The figure shows three views and two pictorial views of one solid part (mm, origin at its lowest corner). Answer the questions. A direction names the side the tool comes from. Coordinates: 2 decimals unless noted, no trailing zeros. Loops run counter-clockwise (first coordinate to the right, second up) from the corner with the lowest first, then second, coordinate; pieces in that order, holes last. Notation, with made-up numbers: M 70,54.5 L 106,54.5 A24 cw 106,92.5 Z; hole C 58.5,69.25 d5. An arc over 180 degrees is marked long. Answer as a JSON object with one key per item and string values. Group by question number.
1. A cutting plane is placed at A-A on x = 10. Give the vertices of the cut face in (y, z), and give its area (3 significant figures).
2. A cutting plane is placed at B-B on z = 2.75. Give the vertices of the cut face in (x, y).
3. For the marked faces 1 and 2, determine the directions among +Z, -Z, +X, -X, +Y, -Y from which every point of the face is accessible in a straight line to the end or side of a thin tool.
4. A cutting plane is placed at D-D on x = 12.5. Give the vertices of the cut face in (y, z).
5. Given pin 1 (6 mm diameter, centred on x = 7.5, y = 23, fed in from -Z); pin 2 (1 mm diameter, centred on x = 4, z = 21.5, fed in from +Y); pin 3 (3 mm diameter, centred on x = 13, y = 40, fed in from +Z), each flat-ended and moving along its own axis, determine where each tip first touches the part or whether it passes through.
6. A cutting plane is placed at C-C on y = 32. Give the vertices of the cut face in (x, z), and give its area (3 significant figures).
7. Straight lines are drawn through the part: L1, parallel to Z at x = 11, y = 3; L2, parallel to X at y = 35, z = 6.75; L3, parallel to X at y = 36, z = 5.25. For each, find the intervals that lie inside material, in ascending order.
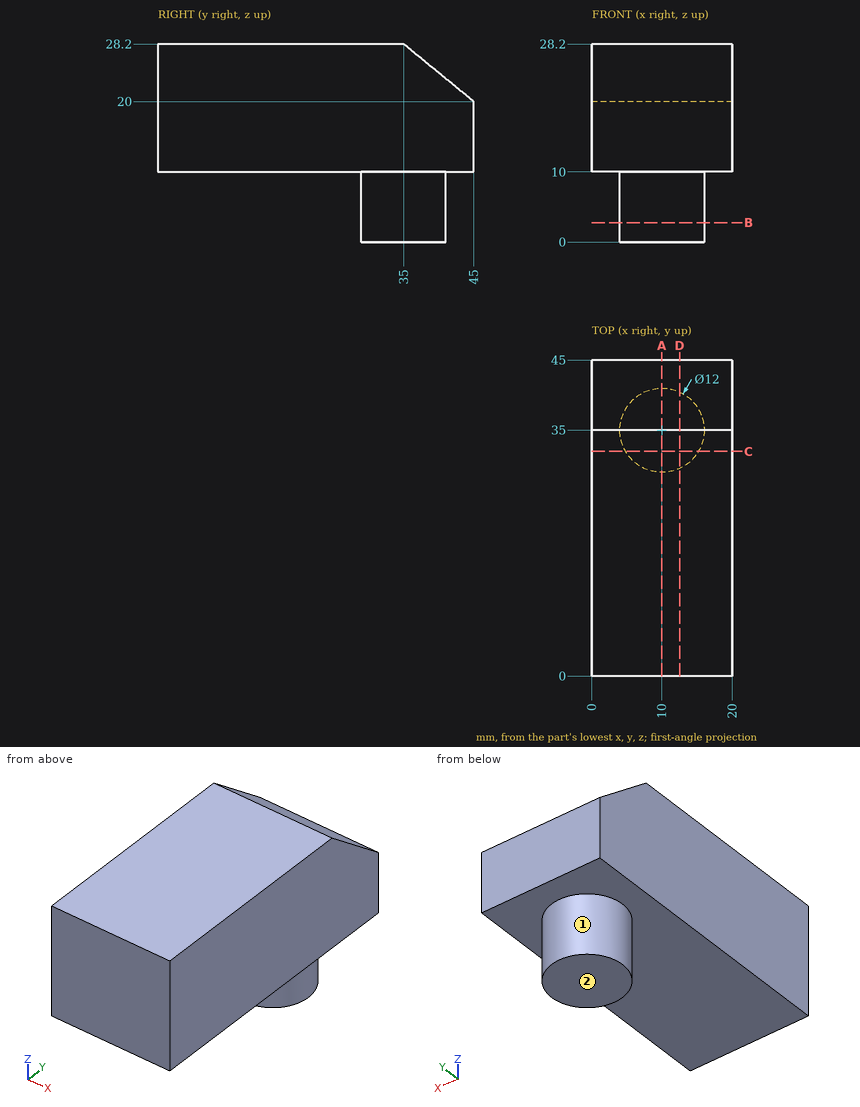
From the geometry:
{
 "1": {"outline": "M 0,10 L 29,10 L 29,0 L 41,0 L 41,10 L 45,10 L 45,20 L 35,28.2 L 0,28.2 Z", "area": "898 mm²"},
 "2": {"outline": "C 10,35 d12"},
 "3": {"face 1": "-Z", "face 2": "-Z, +X, -X, +Y, -Y"},
 "4": {"outline": "M 0,10 L 29.55,10 L 29.55,0 L 40.45,0 L 40.45,10 L 45,10 L 45,20 L 35,28.2 L 0,28.2 Z"},
 "5": {"pin 1": "stops at z = 10", "pin 2": "stops at y = 43.78", "pin 3": "stops at z = 25.33"},
 "6": {"outline": "M 0,10 L 4.8,10 L 4.8,0 L 15.2,0 L 15.2,10 L 20,10 L 20,28.2 L 0,28.2 Z", "area": "468 mm²"},
 "7": {"L1": "z = 10 to 28.2", "L2": "x = 4 to 16", "L3": "x = 4.08 to 15.92"}
}
